For this review, take the finished solid that the model builds, in its own axes (mm). Face numbers are marked on the shaded views. Coordinates: 2 decimals unless noted, no trailing zeros. Loops run counter-clockwise (first coordinate to the right, second up) from the corner with the lowest first, then second, coordinate; pieces in that order, holes last. Notation, with made-up numbers: (-33, -26.75) -> (4, -26.75) arc R17 cw to (4, 5.25) -> close; hole circle Ø8 at (-23, -4.75). An arc over 180 degrees is marked (long way). Answer in a Markdown table with one row per item.
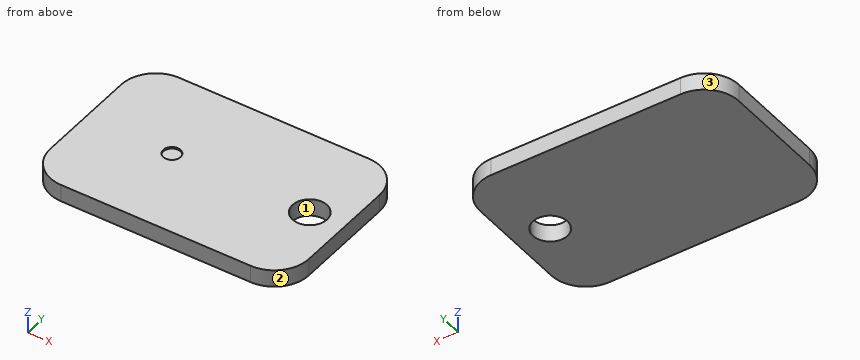
Autodesk Inventor part; units mm, degrees
ref_plane "YZ Plane" through (0, 0, 0) normal (1, 0, 0) x (0, 1, 0)
ref_plane "XZ Plane" through (0, 0, 0) normal (0, 1, 0) x (-1, 0, 0)
ref_plane "XY Plane" through (0, 0, 0) normal (0, 0, 1) x (1, 0, 0)
sketch "Sketch1" plane through (0, 0, 0) normal (0, 0, 1) x (1, 0, 0)
  line L0 (-75, -50) -> (75, -50)
  line L1 (75, -50) -> (75, 50)
  line L2 (75, 50) -> (-75, 50)
  line L3 (-75, 50) -> (-75, -50)
  line L4 (-75, -50) -> (75, 50) construction
  line L5 (75, -50) -> (-75, 50) construction
  circle A0 centre (55, -30) radius 10
  circle A1 centre (55, 30) radius 10
  line L6 (0, 0) -> (75, 0) construction
  circle A2 centre (55, 0) radius 10
  dimension "d0" = 150
  dimension "d1" = 100
  dimension "d23" = 20
  dimension "d25" = 20
  dimension "d26" = 20
extrude "Plate1" add sketch "Sketch1" along normal blind 10 contours L3 L2 L1 L0 | A0 | A1
fillet "Corner Round1" radius 20 4 edges at (75, -50, 5) (-75, -50, 5) (-75, 50, 5) (75, 50, 5)
sketch "Sketch5" plane through (0, 0, 10) normal (0, 0, 1) x (1, 0, 0)
  line L0 (55, -50) -> (-55, -50)
  line L1 (-75, -30) -> (-75, 30)
  line L2 (-55, 50) -> (55, 50)
  circle A0 centre (-25, 0) radius 50
  circle A1 centre (-25, 0) radius 5
  point P0 (0, 0)
  dimension "d27" = 10
extrude "Extrusion2" cut sketch "Sketch5" against normal blind 1 contours A1
equation "\"d26\" = d25"
equation "\"d2\" = Thickness"
equation "\"BendReliefDepth\" = 0.5 * Thickness"
equation "\"TransitionRadius\" = BendRadius"
equation "\"JacobiRadiusSize\" = BendRadius"
properties part number "PNS-783 leg floor plate" material "Steel"
Item 1: The part is to be moulded in two halves that separate along X. For the marked faces 1, 2 and 3, say which applies: +X half, -X half, draft (parallel to the pull), parting line (faces both ways), or undercut.
Worked answers:
| item | result |
|---|---|
| face 1 | undercut |
| face 2 | +X half |
| face 3 | -X half |
Item 2: For L1, parallel to Y at x = -25, z = 9.45; L2, parallel to Y at x = 55, z = 7.75; L3, parallel to X at y = 4, z = 5.5, list the stretches that pass through material, from the lowest coordinate up.
Worked answers:
| item | result |
|---|---|
| L1 | -50 to -5, 5 to 50 |
| L2 | -50 to -10, 10 to 50 |
| L3 | -75 to 45.83, 64.17 to 75 |
Item 3: Take a section at B-B, the plane y = 0. State the section outline as (x, z) points, and give its area (3 significant figures).
Worked answers:
| item | result |
|---|---|
| outline | (-75, 0) -> (45, 0) -> (45, 10) -> (-20, 10) -> (-20, 9) -> (-30, 9) -> (-30, 10) -> (-75, 10) -> close; (65, 0) -> (75, 0) -> (75, 10) -> (65, 10) -> close |
| area | 1,290 mm² |
Item 4: Take a section at C-C, the plane y = -40. State the section outline as (x, z) points.
Worked answers:
| item | result |
|---|---|
| outline | (-72.32, 0) -> (72.32, 0) -> (72.32, 10) -> (-72.32, 10) -> close |
Item 5: Take a section at A-A, the plane z = 1.5. State the section outline as (x, y) points.
Worked answers:
| item | result |
|---|---|
| outline | (-75, -30) arc R20 ccw to (-55, -50) -> (55, -50) arc R20 ccw to (75, -30) -> (75, 30) arc R20 ccw to (55, 50) -> (-55, 50) arc R20 ccw to (-75, 30) -> close; hole circle Ø20 at (55, 0) |
Item 6: Insertion check: pin 1 (9 mm diameter, centred on x = -25, y = 0, fed in from -Z); pin 2 (3 mm diameter, centred on x = -25, y = 1, fed in from +Z). Each pin has a flat end and moves straight along its axis. Give the tip position at first contact, or say it passes through.
Worked answers:
| item | result |
|---|---|
| pin 1 | z = 0 |
| pin 2 | z = 9 |
